Work out the finished part from the listing and answer in its coordinate system (mm). Face numbers are marked on the shaded views. Coordinates: 2 decimals unless noted, no trailing zeros. Write each loop counter-clockwise with the first axis right and the second up, starting at its lowest first coordinate (ties: lowest second). Pieces come first, ordered by that corner, then holes. Notation, with made-up numbers: (-8, -6.5) - (-4, -6.5) arc R11 cw to (-4, 12.5) - close; hole circle Ø1 at (-39, 30). An arc over 180 degrees is marked (long way). Answer as a JSON object with one key per item and string values. Group by question number.
from build123d import *

# Parameters (mm, degrees)
F0_R     = 11.5
F0_R_2   = 4
F1_DEPTH = 30
F2_SIZE  = 1


with BuildPart() as f1:
    # F0 (on Top) → F1 (new body)
    with BuildSketch(Plane.XY):
        Circle(F0_R)
        Circle(F0_R_2, mode=Mode.SUBTRACT)
    extrude(amount=F1_DEPTH)

    # F2
    f2_edges = [f1.edges().sort_by_distance(p)[0] for p in [
        (-4, 0, 30),
        (-11.5, 0, 30),
        (-4, 0, 0),
        (11.5, 0, 15),
        (-11.5, 0, 0),
    ]]
    chamfer(f2_edges, length=F2_SIZE)


solid = f1.part
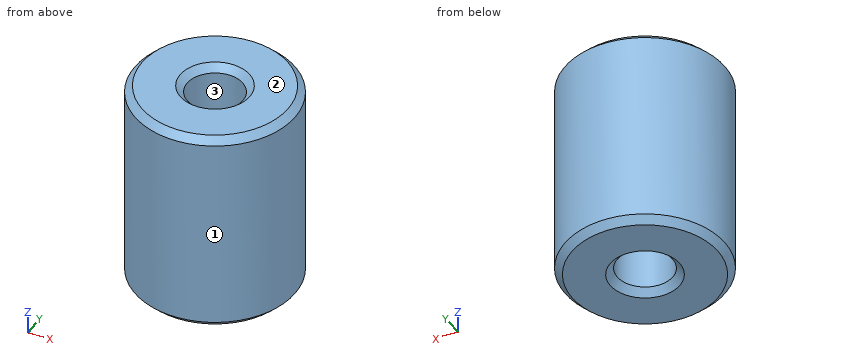
Q1. Consider L1, parallel to Y at x = 0, z = 18.5; L2, parallel to X at y = -0.25, z = 16.75; L3, parallel to X at y = -2.25, z = 12.5. Determine where each line is inside the solid, lowest interval first. Write a range as from..to.
Q2. Flat-ended cylindrical pins translate along their axes: pin 1 Ø6 at (y, z) = (8, 17) entering from -X; pin 2 Ø6 at (x, z) = (-4.5, 11) entering from -Y; pin 3 Ø1 at (y, z) = (-1.5, 18.5) entering from -X. Find the tip coordinate at first contact, or state that the pin passes through.
Q3. Section C-C on z = 7 is taken. Determine the outline of the cut face in (x, y), plus the area to 3 significant figures.
Q4. For a pull along X with two mould halves and no side action, classify the marked faces 1, 2 and 3 as +X half, -X half, draft (parallel to the pull), parting line (faces both ways), or undercut.
Q5. Section A-A on y = 0 is taken. Determine the outline of the cut face in (x, z), plus the area to 3 significant figures.
Numbers:
{
 "1": {"L1": "y = -11.5..-4, 4..11.5", "L2": "x = -11.5..-3.99, 3.99..11.5", "L3": "x = -11.28..-3.31, 3.31..11.28"},
 "2": {"pin 1": "stops at x = -10.36", "pin 2": "stops at y = -11.4", "pin 3": "stops at x = -11.46"},
 "3": {"outline": "circle Ø23 at (0, 0); hole circle Ø8 at (0, 0)", "area": "365 mm²"},
 "4": {"face 1": "parting line", "face 2": "draft", "face 3": "undercut"},
 "5": {"outline": "(-11.5, 1) - (-10.5, 0) - (-5, 0) - (-4, 1) - (-4, 29) - (-5, 30) - (-10.5, 30) - (-11.5, 29) - close; (4, 1) - (5, 0) - (10.5, 0) - (11.5, 1) - (11.5, 29) - (10.5, 30) - (5, 30) - (4, 29) - close", "area": "446 mm²"}
}
